Read the model definition and answer for the solid it produces. Units are mm, in the model's axes. Face numbers are marked on the shaded views. A direction names the side the tool comes from. Coordinates: 2 decimals unless noted, no trailing zeros. Loops run counter-clockwise (first coordinate to the right, second up) from the corner with the lowest first, then second, coordinate; pieces in that order, holes last. Notation, with made-up numbers: (-8, 47) -> (19, 47) arc R8 cw to (19, 56) -> close; hole circle Ø9 at (-25.75, -2). An arc over 180 degrees is marked (long way). Answer in a Markdown table with one row per item.
```python
from build123d import *

# Parameters (mm, degrees)
F1_DEPTH = 13
F3_DEPTH = 25
F4_R     = 2.5
F5_DEPTH = 25
F6_SIZE  = 5


with BuildPart() as f1:
    # F0 (on Front) → F1 (new body)
    with BuildSketch(Plane.XZ):
        Polygon((0, -3.5), (0, 0), (-36, 0), (-36, 36), (-39.5, 36), (-39.5, -3.5), align=None)
    extrude(amount=F1_DEPTH)

    # F2 (on face) → F3 (cut)
    with BuildSketch(Plane.YZ.offset(-36)):
        with BuildLine():
            ThreePointArc((-9, 28.5), (-6.5, 26), (-4, 28.5))
            ThreePointArc((-4, 28.5), (-6.5, 31), (-9, 28.5))
        make_face()
        with BuildLine():
            Line((-4, 12), (-4, 28.5))
            ThreePointArc((-4, 28.5), (-6.5, 26), (-9, 28.5))
            Line((-9, 28.5), (-9, 12))
            ThreePointArc((-9, 12), (-6.5, 14.5), (-4, 12))
        make_face()
        with BuildLine():
            ThreePointArc((-9, 12), (-6.5, 9.5), (-4, 12))
            ThreePointArc((-4, 12), (-6.5, 14.5), (-9, 12))
        make_face()
    extrude(amount=-F3_DEPTH, mode=Mode.SUBTRACT)

    # F4 (on face) → F5 (cut)
    with BuildSketch(Plane.XY):
        with Locations((-7.483315, -6)):
            Circle(F4_R)
    extrude(amount=-F5_DEPTH, mode=Mode.SUBTRACT)

    # F6
    f6_edges = [f1.edges().sort_by_distance(p)[0] for p in [
        (-36, -6.5, 0),
    ]]
    chamfer(f6_edges, length=F6_SIZE)


solid = f1.part
```
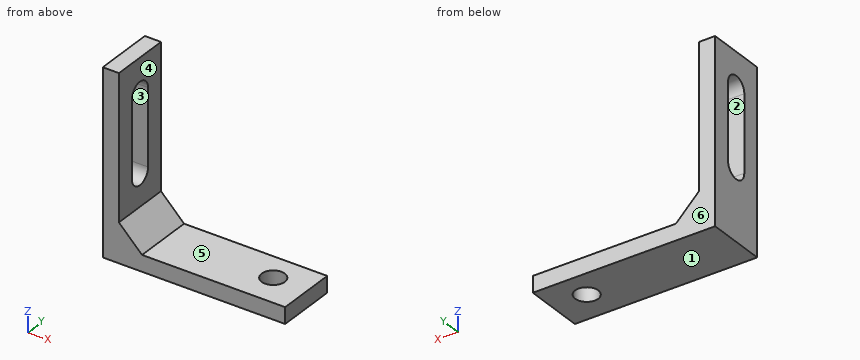
1. A tool of negligible diameter and unlimited length cuts with its end or side. For the marked faces 5 and 6, from which of +Z, -Z, +X, -X, +Y, -Y can it reach the whole face along a straight path? Write none if from no direction.
A:
| item | result |
|---|---|
| face 5 | +Z, +X, +Y, -Y |
| face 6 | +Z, -Z, +X, -X, +Y |
2. A cutting plane is placed at D-D on x = -33. Give the vertices of the cut face in (y, z), and give its area (3 significant figures).
A:
| item | result |
|---|---|
| outline | (-13, -3.5) -> (0, -3.5) -> (0, 2) -> (-13, 2) -> close |
| area | 71.5 mm2 |
3. Given pin 1 Ø6 at (y, z) = (-4, 14.5) entering from +X; pin 2 Ø6 at (x, y) = (-13, -6) entering from +Z; pin 3 Ø2 at (x, y) = (-33, -11.5) entering from +Z, each flat-ended and moving along its own axis, determine where each tip first touches the part or whether it passes through.
A:
| item | result |
|---|---|
| pin 1 | stops at x = -36 |
| pin 2 | stops at z = 0 |
| pin 3 | stops at z = 3 |
4. A cutting plane is placed at B-B on y = -11.5. Give the vertices of the cut face in (x, z).
A:
| item | result |
|---|---|
| outline | (-39.5, -3.5) -> (0, -3.5) -> (0, 0) -> (-31, 0) -> (-36, 5) -> (-36, 36) -> (-39.5, 36) -> close |
5. Find the intervals of material crossed by probe 1 along Z at (x, y) = (-30, -2.5); probe 2 along X at (y, z) = (-3.5, 17.5); probe 3 along Z at (x, y) = (-37, -5), in increasing order.
A:
| item | result |
|---|---|
| probe 1 | z = -3.5 to 0 |
| probe 2 | x = -39.5 to -36 |
| probe 3 | z = -3.5 to 10, 30.5 to 36 |
6. A cutting plane is placed at C-C on y = -5. Give the vertices of the cut face in (x, z), and give its area (3 significant figures).
A:
| item | result |
|---|---|
| outline | (-39.5, -3.5) -> (-9.77, -3.5) -> (-9.77, 0) -> (-31, 0) -> (-36, 5) -> (-36, 10) -> (-39.5, 10) -> close; (-39.5, 30.5) -> (-36, 30.5) -> (-36, 36) -> (-39.5, 36) -> close; (-5.19, -3.5) -> (0, -3.5) -> (0, 0) -> (-5.19, 0) -> close |
| area | 189 mm2 |
7. The mould has two halves that part along Z. Classify the marked faces 1, 2, 3 and 4: pulls with the +Z half, pulls with the -Z half, needs draft (parallel to the pull), parting line crosses it, or undercut.
A:
| item | result |
|---|---|
| face 1 | pulls with the -Z half |
| face 2 | undercut |
| face 3 | undercut |
| face 4 | needs draft |
8. A cutting plane is placed at A-A on z = 13.5. Give the vertices of the cut face in (x, y), and give its area (3 significant figures).
A:
| item | result |
|---|---|
| outline | (-39.5, -13) -> (-36, -13) -> (-36, -9) -> (-39.5, -9) -> close; (-39.5, -4) -> (-36, -4) -> (-36, 0) -> (-39.5, 0) -> close |
| area | 28.0 mm2 |
